CAD build for the part. Positions are in the model's coordinates, mm. Face numbers are marked on the shaded views. A direction names the side the tool comes from. Coordinates: 2 decimals unless noted, no trailing zeros. Write each loop counter-clockwise with the first axis right and the second up, starting at its lowest first coordinate (ties: lowest second). Pieces come first, ordered by that corner, then holes. Notation, with made-up numbers: M 33.25,75 L 52.25,75 A8 cw 52.25,81 Z; hole C 49.5,65.25 d7. An arc over 180 degrees is marked long. Answer as CSV lines item,"result". Start each with the question number.
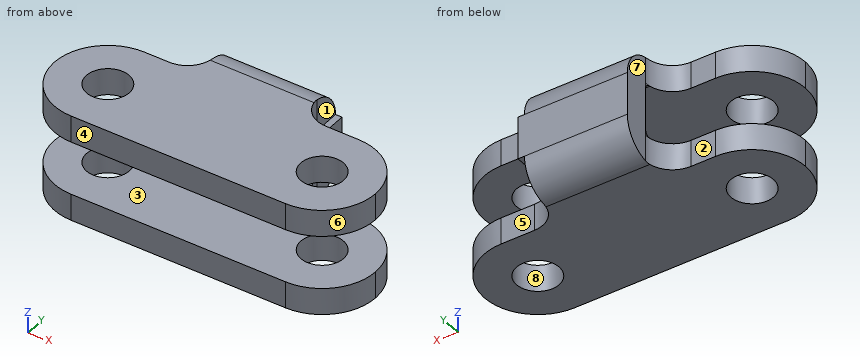
```python
from build123d import *

# Parameters (mm, degrees)
SKETCH1_W           = 38.1
SKETCH1_H           = 19.05
SKETCH1_R           = 2.54
BASE_EXTRUDE_DEPTH  = 12.7
CUT_EXTRUDE1_DEPTH  = 43.121134838
CUT_EXTRUDE2_DEPTH  = 37.477972806
CUT_EXTRUDE3_DEPTH  = 37.477972806
FILLET1_R           = 0.635
FILLET2_R           = 3.81
FILLET3_R           = 6.35
SKETCH6_W           = 5.08
SKETCH6_H           = 3.175
BOSS_EXTRUDE1_DEPTH = 0.762


# Some blends are built 0.0001 mm under size
with BuildPart() as part:
    # Sketch1 → Base-Extrude (new body)
    with BuildSketch(Plane.XY):
        with Locations((12.7, 3.175)):
            Rectangle(SKETCH1_W, SKETCH1_H)
        Circle(SKETCH1_R, mode=Mode.SUBTRACT)
        with Locations((25.4, 0)):
            Circle(SKETCH1_R, mode=Mode.SUBTRACT)
    extrude(amount=-BASE_EXTRUDE_DEPTH)

    # Sketch3 → Cut-Extrude1 (cut, through all)
    with BuildSketch(Plane(origin=(31.75, 0, 0), x_dir=(0, 0, -1), z_dir=(1, 0, 0))):
        Polygon((3.175, -58.947094971), (3.175, -6.35), (3.175, 9.525), (9.525, 9.525), (9.525, -6.35), (9.525, -58.947094971), (9.525, -164.141284914), (3.175, -164.141284914), align=None)
    extrude(amount=-CUT_EXTRUDE1_DEPTH, mode=Mode.SUBTRACT)

    # Sketch4 → Cut-Extrude2 (cut, through all)
    with BuildSketch(Plane.XY):
        with BuildLine():
            Line((-96.671852568, 6.35), (-6.35, 6.35))
            Line((-6.35, 6.35), (2.921, 6.35))
            ThreePointArc((2.921, 6.35), (5.16606403, 7.27993597), (6.096, 9.525))
            Line((6.096, 9.525), (6.096, 12.7))
            Line((6.096, 12.7), (6.096, 103.021852568))
            Line((6.096, 103.021852568), (-117.676302849, 234.599074203))
            Line((-117.676302849, 234.599074203), (-220.444155417, 137.927221634))
            Line((-220.444155417, 137.927221634), (-96.671852568, 6.35))
        make_face()
    extrude(amount=-CUT_EXTRUDE2_DEPTH, mode=Mode.SUBTRACT)

    # Sketch5 → Cut-Extrude3 (cut, through all)
    with BuildSketch(Plane.XY):
        with BuildLine():
            Line((122.071852568, 6.35), (31.75, 6.35))
            Line((31.75, 6.35), (21.463, 6.35))
            ThreePointArc((21.463, 6.35), (19.21793597, 7.27993597), (18.288, 9.525))
            Line((18.288, 9.525), (18.288, 12.7))
            Line((18.288, 12.7), (18.288, 103.021852568))
            Line((18.288, 103.021852568), (141.41301137, 235.20498228))
            Line((141.41301137, 235.20498228), (245.196863939, 138.533129712))
            Line((245.196863939, 138.533129712), (122.071852568, 6.35))
        make_face()
    extrude(amount=-CUT_EXTRUDE3_DEPTH, mode=Mode.SUBTRACT)

    # Fillet1
    # the kernel refuses this fillet: 0.635 mm, written as the material it adds along each edge
    with BuildSketch(Plane(origin=(19.8755, 9.525, -9.525), x_dir=(0, 0, 1), z_dir=(-1, 0, 0))) as fillet1_piece_1_section:
        with BuildLine():
            CenterArc((FILLET1_R, -FILLET1_R), FILLET1_R, 90, 90)
            Line((0, -FILLET1_R), (0, 0))
            Line((0, 0), (FILLET1_R, 0))
        make_face()
    fillet1_piece_1 = extrude(amount=15.367, mode=Mode.PRIVATE)
    fillet1_piece_1 = fillet1_piece_1 - Plane(origin=(2.921, 9.525, -9.486385911), x_dir=(0, -1, 0), z_dir=(0, 0, 1)) * Cylinder(3.175, 34, mode=Mode.PRIVATE)
    fillet1_piece_1 = fillet1_piece_1 - Plane(origin=(21.463, 9.525, -9.486385911), x_dir=(0, -1, 0), z_dir=(0, 0, 1)) * Cylinder(3.175, 34, mode=Mode.PRIVATE)
    add(fillet1_piece_1)
    with BuildSketch(Plane(origin=(19.8755, 9.525, -3.175), x_dir=(0, -1, 0), z_dir=(-1, 0, 0))) as fillet1_piece_2_section:
        with BuildLine():
            CenterArc((FILLET1_R, -FILLET1_R), FILLET1_R, 90, 90)
            Line((0, -FILLET1_R), (0, 0))
            Line((0, 0), (FILLET1_R, 0))
        make_face()
    fillet1_piece_2 = extrude(amount=15.367, mode=Mode.PRIVATE)
    fillet1_piece_2 = fillet1_piece_2 - Plane(origin=(21.463, 9.525, -3.21361614), x_dir=(0, -1, 0), z_dir=(0, 0, 1)) * Cylinder(3.175, 34, mode=Mode.PRIVATE)
    fillet1_piece_2 = fillet1_piece_2 - Plane(origin=(2.921, 9.525, -3.21361614), x_dir=(0, -1, 0), z_dir=(0, 0, 1)) * Cylinder(3.175, 34, mode=Mode.PRIVATE)
    add(fillet1_piece_2)

    # Fillet2
    fillet2_edges = [part.edges().sort_by_distance(p)[0] for p in [
        (12.192, 12.7, 0),
        (12.192, 12.7, -12.7),
    ]]
    fillet(fillet2_edges, radius=FILLET2_R)

    # Fillet3
    fillet3_edges = [part.edges().sort_by_distance(p)[0] for p in [
        (-6.35, -6.35, -1.5875),
        (31.75, -6.35, -1.5875),
        (-6.35, 6.35, -1.5875),
        (-6.35, 6.35, -11.1125),
        (31.75, 6.35, -11.1125),
        (-6.35, -6.35, -11.1125),
        (31.75, 6.35, -1.5875),
        (31.75, -6.35, -11.1125),
    ]]
    fillet(fillet3_edges, radius=FILLET3_R - 0.0001)  # a hair under: the kernel refuses the full size

    # Sketch6 → Boss-Extrude1 (add)
    with BuildSketch(Plane(origin=(18.288, 0, 0), x_dir=(0, 0, -1), z_dir=(1, 0, 0))):
        with Locations((6.35, 11.1125)):
            Rectangle(SKETCH6_W, SKETCH6_H)
    extrude(amount=BOSS_EXTRUDE1_DEPTH)


solid = part.part
```
1) Band-saw the part on B-B, the plane x = 28.5. List the corners of the cut face in (y, z) (3 decimals).
2) Two-plate mould, pull along Y, no slides. Class the marked faces 6, 7 and 8: pulls with the +Y half, pulls with the -Y half, needs draft (parallel to the pull), parting line crosses it, or undercut.
3) Band-saw the part on C-C, the plane z = -11.25. State how many separate pieces and enclosed holes the cut face has, plus the area to 3 significant figures.
4) Probe L1, parallel to Y at x = 25.4, z = -10.8; L2, parallel to Z at x = 8, y = 2.25 (3 decimals); L3, parallel to X at y = 10.5, z = -2.5. List the from-to ranges inside material, lowest first. Write a range as [from, to].
5) Tool access for the marked faces 1, 2, 3, 4 and 5: list every direction of +Z, -Z, +X, -X, +Y, -Y with a clear straight run to the whole face (end or side of a thin tool).
6) Band-saw the part on D-D, the plane x = -3.5. List the corners of the cut face in (y, z) (3 decimals), plus the area to 3 significant figures.
7) Pin check, flat tips, straight feed: P1, Ø0.9, axis at x = 2, z = -11.5, coming from the +Y side; P2, Ø0.6, axis at x = 18.5, y = 10.5, coming from the +Z side; P3, Ø3.5, axis at y = 11, z = -7.5, coming from the +X side. Stop position of each tip, or through.
8) Band-saw the part on A-A, the plane y = -1.5. List the corners of the cut face in (x, z) (3 decimals), plus the area to 3 significant figures.
Result sheet:
1,outline,"M -5.542,-12.7 L 5.542,-12.7 L 5.542,-9.525 L -5.542,-9.525 Z; M -5.542,-3.175 L 5.542,-3.175 L 5.542,0 L -5.542,0 Z"
2,face 6,"pulls with the -Y half"
2,face 7,"needs draft"
2,face 8,"undercut"
3,separate pieces,"1"
3,enclosed holes,"2"
3,area,"480 mm²"
4,L1,"y = [-6.35, -2.54], [2.54, 6.35]"
4,L2,"z = [-12.7, -9.525], [-3.175, 0]"
4,L3,"x = [6.1, 18.29]"
5,face 1,"+Z, +X, +Y"
5,face 2,"+Z, -Z, -X, +Y"
5,face 3,"+X, -X, -Y"
5,face 4,"+Z, -Z, +X, -X, -Y"
5,face 5,"+Z, -Z, +X, +Y"
6,outline,"M -5.298,-12.7 L 5.298,-12.7 L 5.298,-9.525 L -5.298,-9.525 Z; M -5.298,-3.175 L 5.298,-3.175 L 5.298,0 L -5.298,0 Z"
6,area,"67.3 mm²"
7,P1,"stops at y = 6.35"
7,P2,"stops at z = -0.27"
7,P3,"stops at x = 19.05"
8,outline,"M -6.17,-12.7 L -2.05,-12.7 L -2.05,-9.525 L -6.17,-9.525 Z; M -6.17,-3.175 L -2.05,-3.175 L -2.05,0 L -6.17,0 Z; M 2.05,-12.7 L 23.35,-12.7 L 23.35,-9.525 L 2.05,-9.525 Z; M 2.05,-3.175 L 23.35,-3.175 L 23.35,0 L 2.05,0 Z; M 27.45,-12.7 L 31.57,-12.7 L 31.57,-9.525 L 27.45,-9.525 Z; M 27.45,-3.175 L 31.57,-3.175 L 31.57,0 L 27.45,0 Z"
8,area,"188 mm²"
